from build123d import *


with BuildPart() as part:
    # Schizzo1 → Rivoluzione1 (revolve)
    with BuildSketch(Plane.XY):
        with BuildLine():
            Line((-3.8, 3.165), (-3.8, 2.33))
            Line((-3.8, 2.33), (-4, 2.33))
            Line((-4, 2.33), (-4, 1.65))
            Line((-4, 1.65), (-3.85, 1.5))
            Line((-3.85, 1.5), (-0.15, 1.5))
            Line((-0.15, 1.5), (0, 1.65))
            Line((0, 1.65), (0, 2.33))
            Line((0, 2.33), (-0.2, 2.33))
            Line((-0.2, 2.33), (-0.2, 3.165))
            Line((-0.2, 3.165), (0, 3.165))
            Line((0, 3.165), (0, 4.75))
            Line((0, 4.75), (-0.85, 4.75))
            Line((-0.85, 4.75), (-0.85, 4.02))
            ThreePointArc((-0.85, 4.02), (-0.835857864, 3.985857864), (-0.87, 4))
            Line((-0.87, 4), (-3.85, 4))
            Line((-3.85, 4), (-4, 3.85))
            Line((-4, 3.85), (-4, 3.165))
            Line((-4, 3.165), (-3.8, 3.165))
        make_face()
    revolve(axis=Axis((-4, 0, 0), (1, 0, 0)))


solid = part.part
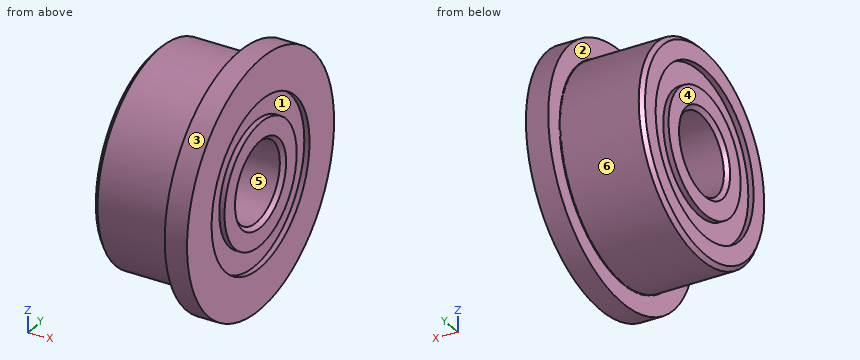
Build history of the part. All positions in model axes, mm. Face numbers are marked on the shaded views. A direction names the side the tool comes from. Round coordinates to 2 decimals unless told otherwise and drop trailing zeros. Loops run counter-clockwise (first coordinate to the right, second up) from the corner with the lowest first, then second, coordinate; pieces in that order, holes last. Notation, with made-up numbers: (87.25, 63) -> (101.25, 63) arc R20 cw to (101.25, 98) -> close; hole circle Ø11 at (-9.75, -4.5). An arc over 180 degrees is marked (long way). One line per item, written item: value. Start each with the question number.
Q1. Two-plate mould, pull along Z, no slides. Class the marked faces 4, 5 and 6: released by +Z, released by -Z, zero draft, split by the parting line, or undercut.
Q2. Probe line 1 along Z through (x, y) = (-2.95, 0); line 2 along X through (y, z) = (-2.25, 2); line 3 along Y through (x, z) = (-1.85, 0.75). List the from-to ranges inside material, lowest first.
Q3. Cut at A-A on x = -2.25. List the corners of the cut face in (y, z).
Q4. 3-axis set-ups, long thin cutter, end or side, ignore diameter. For the marked faces 1, 2 and 3: which of +Z, -Z, +X, -X, +Y, -Y reach the whole face in a straight line?
Q5. Cut at B-B on x = -0.35. List the corners of the cut face in (y, z), plus the area to 3 significant figures.
Q6. Drop flat-ended pins along their axis: pin 1 Ø5.5 at (y, z) = (0, 0) entering from +X; pin 2 Ø2 at (x, y) = (-3, -4) entering from -Z; pin 3 Ø2 at (x, y) = (-2.5, -1.5) entering from +Z; pin 4 Ø1 at (x, y) = (-3, 2) entering from +Z. Give the stop position or say it passes through.
Computed:
1. face 4: zero draft
1. face 5: undercut
1. face 6: split by the parting line
2. line 1: -4 to -1.5, 1.5 to 4
2. line 2: -3.8 to -0.2
2. line 3: -3.93 to -1.3, 1.3 to 3.93
3. outline: circle Ø8 at (0, 0); hole circle Ø3 at (0, 0)
4. face 1: +X
4. face 2: -X
4. face 3: +X, -X
5. outline: circle Ø9.5 at (0, 0); hole circle Ø3 at (0, 0)
5. area: 63.8 mm²
6. pin 1: x = 0
6. pin 2: z = -2.65
6. pin 3: z = 3.97
6. pin 4: z = 3.71
